```python
from build123d import *

# Parameters (mm, degrees)
SKETCH_1_R               = 2
EXTRUDE_1_DEPTH          = 1.5
SKETCH_2_R               = 1
EXTRUDE_2_DEPTH          = 20
CUT_EXTRUDE_1_DEPTH      = 22.685248442
CUT_EXTRUDE_1_DEPTH_BACK = 1
SKETCH_4_W               = 4
SKETCH_4_H               = 0.2
SKETCH_4_W_2             = 0.2
SKETCH_4_H_2             = 4
FILLET_1_R               = 1


with BuildPart() as part:
    # Sketch 1 → Extrude 1 (new body)
    with BuildSketch(Plane(origin=(0, 0, 0), x_dir=(1, 0, 0), z_dir=(0, 1, 0))):
        with Locations(Location((0, 0, 0), (0, 0, 270))):
            Circle(SKETCH_1_R)
    extrude(amount=-EXTRUDE_1_DEPTH)

    # Sketch 2 → Extrude 2 (add)
    with BuildSketch(Plane(origin=(0, 0, 0), x_dir=(1, 0, 0), z_dir=(0, 1, 0))):
        with Locations(Location((0, 0, 0), (0, 0, 270))):
            Circle(SKETCH_2_R)
    extrude(amount=EXTRUDE_2_DEPTH)

    # Sketch 4 → Cut-Extrude 1 (cut, two sides: drawn at the far end of the back side and taken through both)
    with BuildSketch(Plane.XZ.offset(1.5).offset(-CUT_EXTRUDE_1_DEPTH_BACK)):
        Rectangle(SKETCH_4_W, SKETCH_4_H)
        Rectangle(SKETCH_4_W_2, SKETCH_4_H_2)
    extrude(amount=CUT_EXTRUDE_1_DEPTH + CUT_EXTRUDE_1_DEPTH_BACK, mode=Mode.SUBTRACT)

    # Fillet 1
    fillet_1_edges = [part.edges().sort_by_distance(p)[0] for p in [
        (1.414213562, -1.5, 1.414213562),
        (-1.414213562, -1.5, 1.414213562),
        (-1.414213562, -1.5, -1.414213562),
        (1.414213562, -1.5, -1.414213562),
    ]]
    fillet(fillet_1_edges, radius=FILLET_1_R)


solid = part.part
```
Read the model definition and answer for the solid it produces. Units are mm, in the model's axes. A direction names the side the tool comes from. Coordinates: 2 decimals unless noted, no trailing zeros. Order: outer loops, then holes, each group sorted by start corner. A loop starts at its lowest first (then second) coordinate and runs counter-clockwise, first axis right, second up. Notation, with made-up numbers: (-7.75, -26) - (12.25, -26) arc R16 ccw to (12.25, -14) - close; hole circle Ø5 at (31.25, 81). An arc over 180 degrees is marked (long way). Answer as a JSON object with one key per item and string values. Group by question number.
Item 1: Section A-A (y = 2) is taken. Give the vertices of the cut face in (x, z), plus the area to 3 significant figures.
Item 2: Consider probe 1 along X at (y, z) = (10.5, 0.1); probe 2 along Y at (x, z) = (0.05, 1.25); probe 3 along Z at (x, y) = (-0.25, 7.5). Determine where each line is inside the solid, lowest interval first. Write a range as from..to.
Item 3: A tool of negligible diameter and unlimited length cuts with its end or side. For faces 4 (the face through (1, -1, -0.1)), 5 (the face through (-0.1, -1, -1)), 6 (the face through (0, 20, 0)), 7 (the face through (0.5, -1.5, -0.5)), 8 (the face through (-1, 10, 0)), from which of +Z, -Z, +X, -X, +Y, -Y can it reach the whole face along a straight path? Write none if from no direction.
Item 4: The mould has two halves that part along Z. Classify faces 1 (the face through (0.1, -1, 1)), 2 (the face through (-1.952, -0.246, -0.434)), 3 (the face through (-1, -1, -0.1)): +Z half, -Z half, draft (parallel to the pull), parting line (faces both ways), or undercut.
Item 5: Flat-ended cylindrical pins translate along their axes: P1, Ø1.1, axis at y = -1, z = -1, coming from the +X side; P2, Ø0.8, axis at y = -1, z = -1, coming from the -X side; P3, Ø1.1, axis at x = 1.5, y = -1, coming from the -Z side. Find the tip coordinate at first contact, or state that the pin passes through.
Results are:
{
 "1": {"outline": "circle Ø2 at (0, 0)", "area": "3.14 mm^2"},
 "2": {"probe 1": "x = -0.99..0.99", "probe 2": "y = -0.5..0", "probe 3": "z = -0.97..0.97"},
 "3": {"face 4": "+X, -X, -Y", "face 5": "+Z, -Z, -Y", "face 6": "+Z, -Z, +X, -X, +Y", "face 7": "+Z, -Z, +X, -X, -Y", "face 8": "+Y"},
 "4": {"face 1": "draft", "face 2": "parting line", "face 3": "undercut"},
 "5": {"P1": "stops at x = 1.91", "P2": "stops at x = -1.84", "P3": "stops at z = -1.69"}
}
